from build123d import *

# Parameters (mm, degrees)
CROQUIS2_W                   = 140
CROQUIS2_H                   = 35
SALIENTE_EXTRUIR1_DEPTH      = 17.5
SALIENTE_EXTRUIR2_DEPTH      = 15
SALIENTE_EXTRUIR2_DEPTH_BACK = 50
CROQUIS3_W                   = 125
CROQUIS3_H                   = 5
CROQUIS4_R                   = 13
CORTAR_EXTRUIR1_DEPTH        = 140
CROQUIS5_W                   = 50
CROQUIS5_H                   = 21
CORTAR_EXTRUIR2_DEPTH        = 192.605062564


with BuildPart() as part:
    # Croquis2 → Saliente-Extruir1 (new body)
    with BuildSketch(Plane.XY):
        with Locations((0, 145)):
            Rectangle(CROQUIS2_W, CROQUIS2_H)
    extrude(amount=SALIENTE_EXTRUIR1_DEPTH)

    # Croquis3 → Saliente-Extruir2 (add, two sides: drawn at the far end of the back side and taken through both)
    with BuildSketch(Plane.XZ.offset(-127.5).offset(-SALIENTE_EXTRUIR2_DEPTH_BACK)):
        with Locations((0, 2.5)):
            Rectangle(CROQUIS3_W, CROQUIS3_H)
    extrude(amount=SALIENTE_EXTRUIR2_DEPTH + SALIENTE_EXTRUIR2_DEPTH_BACK)

    # Croquis4 → Cortar-Extruir1 (cut)
    with BuildSketch(Plane(origin=(70, 0, 0), x_dir=(0, 0, -1), z_dir=(1, 0, 0))):
        with Locations((0, 145)):
            Circle(CROQUIS4_R)
    extrude(amount=-CORTAR_EXTRUIR1_DEPTH, mode=Mode.SUBTRACT)

    # Croquis5 → Cortar-Extruir2 (cut, through all)
    with BuildSketch(Plane.XY.offset(17.5)):
        with Locations((0, 145)):
            Rectangle(CROQUIS5_W, CROQUIS5_H)
    extrude(amount=-CORTAR_EXTRUIR2_DEPTH, mode=Mode.SUBTRACT)


solid = part.part
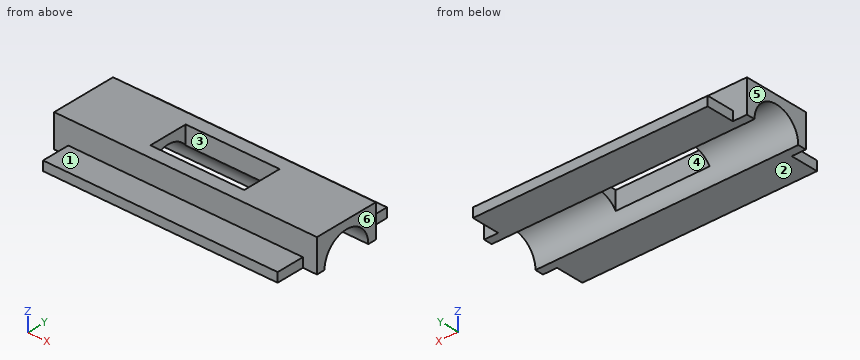
For this review, take the finished solid that the model builds, in its own axes (mm). Face numbers are marked on the shaded views. A direction names the side the tool comes from. Round coordinates to 2 decimals unless told otherwise and drop trailing zeros. Write each loop counter-clockwise with the first axis right and the second up, starting at its lowest first coordinate (ties: lowest second). Pieces come first, ordered by that corner, then holes. Notation, with made-up numbers: (87, 82) -> (106, 82) arc R16 cw to (106, 101) -> close; hole circle Ø4 at (38.5, 31). An arc over 180 degrees is marked (long way). Put each result on its own line as item: value.
Q1. Clearance check with flat-ended pins moving along their axes: pin 1 Ø2 at (y, z) = (120.5, 5) entering from -X; pin 2 Ø5.5 at (y, z) = (171.5, 3) entering from +X; pin 3 Ø4.5 at (x, y) = (-25.5, 117) entering from +Z. State where each tip first meets the part, or that it passes through.
Determined:
pin 1: stops at x = -62.5
pin 2: stops at x = 62.5
pin 3: stops at z = 5
Q2. Machinability: for the marked faces 1, 2 and 3, which of the approach directions +Z, -Z, +X, -X, +Y, -Y give a long, thin tool a straight path to every point of the face, cutting with its end or side? Answer none if there is none.
Determined:
face 1: +Z, +X, -X, -Y
face 2: -Z, +X, -X, +Y, -Y
face 3: +Z, -Z
Q3. Consider section B-B on y = 145. State the section outline as (x, z) points, and give its area (3 significant figures).
Determined:
outline: (-70, 13) -> (-25, 13) -> (-25, 17.5) -> (-70, 17.5) -> close; (25, 13) -> (70, 13) -> (70, 17.5) -> (25, 17.5) -> close
area: 405 mm^2
Q4. To check wall thickness, follow L1, parallel to Y at x = -14.5, z = 9.5; L2, parallel to X at y = 147, z = 16; L3, parallel to X at y = 118, z = 1. State the ranges of each line that lie inside material, in increasing order. Write a range as [from, to].
Determined:
L1: y = [127.5, 134.5], [155.5, 162.5]
L2: x = [-70, -25], [25, 70]
L3: x = [-62.5, 62.5]
Q5. Consider section A-A on x = -5.5. State the section outline as (y, z) points.
Determined:
outline: (112.5, 0) -> (132, 0) arc R13 cw to (134.5, 7.66) -> (134.5, 17.5) -> (127.5, 17.5) -> (127.5, 5) -> (112.5, 5) -> close; (155.5, 7.66) arc R13 cw to (158, 0) -> (177.5, 0) -> (177.5, 5) -> (162.5, 5) -> (162.5, 17.5) -> (155.5, 17.5) -> close
Q6. The part is to be moulded in two halves that separate along X. For the marked faces 4, 5 and 6, say which applies: released by +X, released by -X, zero draft, split by the parting line, or undercut.
Determined:
face 4: undercut
face 5: released by -X
face 6: released by +X
Q7. Consider section C-C on x = -30. State the section outline as (y, z) points, and give its area (3 significant figures).
Determined:
outline: (112.5, 0) -> (132, 0) arc R13 cw to (158, 0) -> (177.5, 0) -> (177.5, 5) -> (162.5, 5) -> (162.5, 17.5) -> (127.5, 17.5) -> (127.5, 5) -> (112.5, 5) -> close
area: 497 mm^2
Q8. Consider section D-D on y = 152. State the section outline as (x, z) points.
Determined:
outline: (-70, 10.95) -> (-25, 10.95) -> (-25, 17.5) -> (-70, 17.5) -> close; (25, 10.95) -> (70, 10.95) -> (70, 17.5) -> (25, 17.5) -> close
